from build123d import *

# Parameters (mm, degrees)
F0_R     = 1.5
F0_W     = 40
F0_H     = 10
F0_W_2   = 15
F0_H_2   = 5
F0_W_3   = 36
F0_H_3   = 40
F0_H_4   = 24
F1_DEPTH = 4


# Not quite as in the source:
# - a feature names something its author has since deleted; it is built from what else it names


with BuildPart() as f1:
    # F0 (on Top) → F1 (new body)
    with BuildSketch(Plane.XY):
        Polygon((-46.7653718044, -100), (46.7653718044, -100), (63.2198544763, -90.5), (109.9852262806, -9.5), (109.9852262806, 9.5), (63.2198544763, 90.5), (46.7653718044, 100), (-46.7653718044, 100), (-54.9926131403, 95.25), (-63.2198544763, 90.5), (-109.9852262806, 9.5), (-109.9852262806, -9.5), (-63.2198544763, -90.5), align=None)
        with Locations((-58.5547909668, -87.4198729811)):
            Circle(F0_R, mode=Mode.SUBTRACT)
        with Locations((-67.5, -61.6776695297)):
            Circle(F0_R, mode=Mode.SUBTRACT)
        with Locations((-46.4304353138, -94.4198729811)):
            Circle(F0_R, mode=Mode.SUBTRACT)
        with Locations((-38.4304353138, -80.5634665205)):
            Circle(F0_R, mode=Mode.SUBTRACT)
        with Locations((-50.5547909668, -73.5634665205)):
            Circle(F0_R, mode=Mode.SUBTRACT)
        with Locations((-85.1776695297, -44)):
            Circle(F0_R, mode=Mode.SUBTRACT)
        with Locations((46.4304353138, -94.4198729811)):
            Circle(F0_R, mode=Mode.SUBTRACT)
        with Locations((38.4304353138, -80.5634665205)):
            Circle(F0_R, mode=Mode.SUBTRACT)
        with Locations((0, -75)):
            Rectangle(F0_W, F0_H, mode=Mode.SUBTRACT)
        with Locations((50.5547909668, -73.5634665205)):
            Circle(F0_R, mode=Mode.SUBTRACT)
        with Locations((58.5547909668, -87.4198729811)):
            Circle(F0_R, mode=Mode.SUBTRACT)
        with Locations((67.5, -61.6776695297)):
            Circle(F0_R, mode=Mode.SUBTRACT)
        with Locations((85.1776695297, -44)):
            Circle(F0_R, mode=Mode.SUBTRACT)
        with Locations((88.9852262806, -7)):
            Circle(F0_R, mode=Mode.SUBTRACT)
        with Locations((104.9852262806, -7)):
            Circle(F0_R, mode=Mode.SUBTRACT)
        with BuildLine():
            Line((-90.4852262806, -7), (-103.4852262806, -7))
            ThreePointArc((-103.4852262806, -7), (-106.0458864524, -8.0606601718), (-104.9852262806, -5.5))
            Line((-104.9852262806, -5.5), (-104.9852262806, 5.5))
            ThreePointArc((-104.9852262806, 5.5), (-106.0458864524, 8.0606601718), (-103.4852262806, 7))
            Line((-103.4852262806, 7), (-90.4852262806, 7))
            ThreePointArc((-90.4852262806, 7), (-88.9852262806, 8.5), (-87.4852262806, 7))
            ThreePointArc((-87.4852262806, 7), (-87.9245661088, 5.9393398282), (-88.9852262806, 5.5))
            Line((-88.9852262806, 5.5), (-88.9852262806, -5.5))
            ThreePointArc((-88.9852262806, -5.5), (-87.9245661088, -5.9393398282), (-87.4852262806, -7))
            ThreePointArc((-87.4852262806, -7), (-88.9852262806, -8.5), (-90.4852262806, -7))
        make_face(mode=Mode.SUBTRACT)
        with BuildLine():
            Line((-48.3223304703, 44), (-18, 44))
            Line((-18, 44), (-18, 52))
            Line((-18, 52), (-7.5, 52))
            Line((-7.5, 52), (-7.5, 57))
            Line((-7.5, 57), (7.5, 57))
            Line((7.5, 57), (7.5, 52))
            Line((7.5, 52), (18, 52))
            Line((18, 52), (18, 44))
            Line((18, 44), (48.3223304703, 44))
            ThreePointArc((48.3223304703, 44), (49.8223304703, 45.5), (51.3223304703, 44))
            Line((51.3223304703, 44), (67.5, 44))
            Line((67.5, 44), (67.5, 27.8223304703))
            ThreePointArc((67.5, 27.8223304703), (68.5606601718, 27.3829906421), (69, 26.3223304703))
            ThreePointArc((69, 26.3223304703), (68.5606601718, 25.2616702986), (67.5, 24.8223304703))
            Line((67.5, 24.8223304703), (67.5, -24.8223304703))
            ThreePointArc((67.5, -24.8223304703), (68.5606601718, -25.2616702986), (69, -26.3223304703))
            ThreePointArc((69, -26.3223304703), (68.5606601718, -27.3829906421), (67.5, -27.8223304703))
            Line((67.5, -27.8223304703), (67.5, -44))
            Line((67.5, -44), (51.3223304703, -44))
            ThreePointArc((51.3223304703, -44), (49.8223304703, -45.5), (48.3223304703, -44))
            Line((48.3223304703, -44), (18, -44))
            Line((18, -44), (18, -52))
            Line((18, -52), (7.5, -52))
            Line((7.5, -52), (7.5, -57))
            Line((7.5, -57), (-7.5, -57))
            Line((-7.5, -57), (-7.5, -52))
            Line((-7.5, -52), (-18, -52))
            Line((-18, -52), (-18, -44))
            Line((-18, -44), (-48.3223304703, -44))
            ThreePointArc((-48.3223304703, -44), (-49.8223304703, -45.5), (-51.3223304703, -44))
            Line((-51.3223304703, -44), (-67.5, -44))
            Line((-67.5, -44), (-67.5, -27.8223304703))
            ThreePointArc((-67.5, -27.8223304703), (-69, -26.3223304703), (-67.5, -24.8223304703))
            Line((-67.5, -24.8223304703), (-67.5, 24.8223304703))
            ThreePointArc((-67.5, 24.8223304703), (-68.8858192988, 25.7483053218), (-68.5606601718, 27.3829906421))
            Line((-68.5606601718, 27.3829906421), (-84.1170093579, 42.9393398282))
            ThreePointArc((-84.1170093579, 42.9393398282), (-86.6776695297, 44), (-84.1170093579, 45.0606601718))
            Line((-84.1170093579, 45.0606601718), (-68.5606601718, 60.6170093579))
            ThreePointArc((-68.5606601718, 60.6170093579), (-68.0740251485, 63.0634888284), (-66, 61.6776695297))
            ThreePointArc((-66, 61.6776695297), (-66.1141807012, 61.1036443811), (-66.4393398282, 60.6170093579))
            Line((-66.4393398282, 60.6170093579), (-50.8829906421, 45.0606601718))
            ThreePointArc((-50.8829906421, 45.0606601718), (-49.2483053218, 45.3858192988), (-48.3223304703, 44))
        make_face(mode=Mode.SUBTRACT)
        with Locations((-58.5547909668, 87.4198729811)):
            Circle(F0_R, mode=Mode.SUBTRACT)
        with Locations((-50.5547909668, 73.5634665205)):
            Circle(F0_R, mode=Mode.SUBTRACT)
        with Locations((-38.4304353138, 80.5634665205)):
            Circle(F0_R, mode=Mode.SUBTRACT)
        with Locations((-46.4304353138, 94.4198729811)):
            Circle(F0_R, mode=Mode.SUBTRACT)
        with Locations((88.9852262806, 7)):
            Circle(F0_R, mode=Mode.SUBTRACT)
        with Locations((104.9852262806, 7)):
            Circle(F0_R, mode=Mode.SUBTRACT)
        with Locations((85.1776695297, 44)):
            Circle(F0_R, mode=Mode.SUBTRACT)
        with Locations((50.5547909668, 73.5634665205)):
            Circle(F0_R, mode=Mode.SUBTRACT)
        with Locations((0, 75)):
            Rectangle(F0_W, F0_H, mode=Mode.SUBTRACT)
        with Locations((38.4304353138, 80.5634665205)):
            Circle(F0_R, mode=Mode.SUBTRACT)
        with Locations((46.4304353138, 94.4198729811)):
            Circle(F0_R, mode=Mode.SUBTRACT)
        with Locations((67.5, 61.6776695297)):
            Circle(F0_R, mode=Mode.SUBTRACT)
        with Locations((58.5547909668, 87.4198729811)):
            Circle(F0_R, mode=Mode.SUBTRACT)
        with BuildLine():
            Line((21, 20), (18, 20))
            Line((18, 20), (18, -20))
            Line((18, -20), (21, -20))
            ThreePointArc((21, -20), (21.4393398282, -18.9393398282), (22.5, -18.5))
            Line((22.5, -18.5), (22.5, 18.5))
            ThreePointArc((22.5, 18.5), (21.4393398282, 18.9393398282), (21, 20))
        make_face()
        Polygon((-18, 52), (-18, 44), (18, 44), (18, 52), (7.5, 52), (7.5, 47), (-7.5, 47), (-7.5, 52), align=None)
        with Locations((0, 49.5)):
            Rectangle(F0_W_2, F0_H_2)
        with BuildLine():
            Line((-18, 20), (-21, 20))
            ThreePointArc((-21, 20), (-21.4393398282, 18.9393398282), (-22.5, 18.5))
            Line((-22.5, 18.5), (-22.5, -18.5))
            ThreePointArc((-22.5, -18.5), (-21.4393398282, -18.9393398282), (-21, -20))
            Line((-21, -20), (-18, -20))
            Line((-18, -20), (-18, 20))
        make_face()
        Polygon((18, -44), (-18, -44), (-18, -52), (-7.5, -52), (-7.5, -47), (7.5, -47), (7.5, -52), (18, -52), align=None)
        Rectangle(F0_W_3, F0_H_3)
        with Locations((0, -49.5)):
            Rectangle(F0_W_2, F0_H_2)
        with BuildLine():
            ThreePointArc((-22.5, 18.5), (-23.5606601718, 21.0606601718), (-21, 20))
            Line((-21, 20), (-18, 20))
            Line((-18, 20), (-18, 44))
            Line((-18, 44), (-48.3223304703, 44))
            ThreePointArc((-48.3223304703, 44), (-49.2483053218, 42.6141807012), (-50.8829906421, 42.9393398282))
            Line((-50.8829906421, 42.9393398282), (-66.4393398282, 27.3829906421))
            ThreePointArc((-66.4393398282, 27.3829906421), (-66.1141807012, 26.8963556189), (-66, 26.3223304703))
            ThreePointArc((-66, 26.3223304703), (-66.4393398282, 25.2616702986), (-67.5, 24.8223304703))
            Line((-67.5, 24.8223304703), (-67.5, -24.8223304703))
            ThreePointArc((-67.5, -24.8223304703), (-66.4393398282, -25.2616702986), (-66, -26.3223304703))
            ThreePointArc((-66, -26.3223304703), (-66.4393398282, -27.3829906421), (-67.5, -27.8223304703))
            Line((-67.5, -27.8223304703), (-67.5, -44))
            Line((-67.5, -44), (-51.3223304703, -44))
            ThreePointArc((-51.3223304703, -44), (-49.8223304703, -42.5), (-48.3223304703, -44))
            Line((-48.3223304703, -44), (-18, -44))
            Line((-18, -44), (-18, -20))
            Line((-18, -20), (-21, -20))
            ThreePointArc((-21, -20), (-23.5606601718, -21.0606601718), (-22.5, -18.5))
            Line((-22.5, -18.5), (-22.5, 18.5))
        make_face()
        with BuildLine():
            ThreePointArc((-51.3223304703, 44), (-51.2081497691, 44.5740251485), (-50.8829906421, 45.0606601718))
            Line((-50.8829906421, 45.0606601718), (-66.4393398282, 60.6170093579))
            ThreePointArc((-66.4393398282, 60.6170093579), (-67.5, 60.1776695297), (-68.5606601718, 60.6170093579))
            Line((-68.5606601718, 60.6170093579), (-84.1170093579, 45.0606601718))
            ThreePointArc((-84.1170093579, 45.0606601718), (-83.7918502309, 44.5740251485), (-83.6776695297, 44))
            ThreePointArc((-83.6776695297, 44), (-83.7918502309, 43.4259748515), (-84.1170093579, 42.9393398282))
            Line((-84.1170093579, 42.9393398282), (-68.5606601718, 27.3829906421))
            ThreePointArc((-68.5606601718, 27.3829906421), (-68.0740251485, 27.7081497691), (-67.5, 27.8223304703))
            Line((-67.5, 27.8223304703), (-67.5, 44))
            Line((-67.5, 44), (-51.3223304703, 44))
        make_face()
        with BuildLine():
            Line((-66.4393398282, 27.3829906421), (-50.8829906421, 42.9393398282))
            ThreePointArc((-50.8829906421, 42.9393398282), (-51.2081497691, 43.4259748515), (-51.3223304703, 44))
            Line((-51.3223304703, 44), (-67.5, 44))
            Line((-67.5, 44), (-67.5, 27.8223304703))
            ThreePointArc((-67.5, 27.8223304703), (-66.9259748515, 27.7081497691), (-66.4393398282, 27.3829906421))
        make_face()
        with BuildLine():
            Line((18, 44), (18, 20))
            Line((18, 20), (21, 20))
            ThreePointArc((21, 20), (22.5, 21.5), (24, 20))
            ThreePointArc((24, 20), (23.5606601718, 18.9393398282), (22.5, 18.5))
            Line((22.5, 18.5), (22.5, -18.5))
            ThreePointArc((22.5, -18.5), (23.5606601718, -18.9393398282), (24, -20))
            ThreePointArc((24, -20), (22.5, -21.5), (21, -20))
            Line((21, -20), (18, -20))
            Line((18, -20), (18, -44))
            Line((18, -44), (48.3223304703, -44))
            ThreePointArc((48.3223304703, -44), (49.8223304703, -42.5), (51.3223304703, -44))
            Line((51.3223304703, -44), (67.5, -44))
            Line((67.5, -44), (67.5, -27.8223304703))
            ThreePointArc((67.5, -27.8223304703), (66, -26.3223304703), (67.5, -24.8223304703))
            Line((67.5, -24.8223304703), (67.5, 24.8223304703))
            ThreePointArc((67.5, 24.8223304703), (66, 26.3223304703), (67.5, 27.8223304703))
            Line((67.5, 27.8223304703), (67.5, 44))
            Line((67.5, 44), (51.3223304703, 44))
            ThreePointArc((51.3223304703, 44), (49.8223304703, 42.5), (48.3223304703, 44))
            Line((48.3223304703, 44), (18, 44))
        make_face()
        with Locations((0, 32)):
            Rectangle(F0_W_3, F0_H_4)
        with Locations((0, -32)):
            Rectangle(F0_W_3, F0_H_4)
        with BuildLine():
            ThreePointArc((-104.9852262806, -5.5), (-103.9245661088, -5.9393398282), (-103.4852262806, -7))
            Line((-103.4852262806, -7), (-90.4852262806, -7))
            ThreePointArc((-90.4852262806, -7), (-90.0458864524, -5.9393398282), (-88.9852262806, -5.5))
            Line((-88.9852262806, -5.5), (-88.9852262806, 5.5))
            ThreePointArc((-88.9852262806, 5.5), (-90.0458864524, 5.9393398282), (-90.4852262806, 7))
            Line((-90.4852262806, 7), (-103.4852262806, 7))
            ThreePointArc((-103.4852262806, 7), (-103.9245661088, 5.9393398282), (-104.9852262806, 5.5))
            Line((-104.9852262806, 5.5), (-104.9852262806, -5.5))
        make_face()
    extrude(amount=F1_DEPTH)


solid = f1.part
The listing builds one solid part. Answer for the finished solid, in the listing's coordinates (mm). Coordinates: 2 decimals unless noted, no trailing zeros. Loops run counter-clockwise (first coordinate to the right, second up) from the corner with the lowest first, then second, coordinate; pieces in that order, holes last.
1) Find the intervals of material crossed by L1, parallel to Y at x = 10.5, z = 3; L2, parallel to Y at x = -67.5, z = 1.3; L3, parallel to X at y = 88, z = 1.95, in increasing order.
2) Flat-ended cylindrical pins translate along their axes: pin 1 Ø1.5 at (x, z) = (-72, 2.5) entering from +Y; pin 2 Ø1 at (y, z) = (63, 3.5) entering from -X; pin 3 Ø1.5 at (x, z) = (51, 2.5) entering from +Y. Find the tip coordinate at first contact, or state that the pin passes through.
3) Find section A-A on z = 1.6. Give the number of separate pieces and of enclosed holes in the cut face, then the cut area to 3 significant figures.
4) Find section B-B on x = 77.5. Write down the section's boundary in (y, z).
Values:
1. L1: y = -100 to -80, -70 to 70, 80 to 100
1. L2: y = -83.09 to -63.18, -60.18 to -27.82, -24.82 to 24.82, 27.82 to 60.18, 63.18 to 83.09
1. L3: x = -64.66 to -59.94, -57.17 to 57.17, 59.94 to 64.66
2. pin 1: stops at y = 76.59
2. pin 2: stops at x = -79.39
2. pin 3: stops at y = 97.99
3. separate pieces: 1
3. enclosed holes: 48
3. area: 33,100 mm2
4. outline: (-65.77, 0) - (65.77, 0) - (65.77, 4) - (-65.77, 4) - close
